Source: CAD feature listing. Evaluate the final solid. Frame: model axes, mm. Round coordinates to 2 decimals unless told otherwise and drop trailing zeros. Order: outer loops, then holes, each group sorted by start corner. A loop starts at its lowest first (then second) coordinate and runs counter-clockwise, first axis right, second up. Notation, with made-up numbers: (20, 81.5) -> (29, 81.5) arc R21 ccw to (29, 93.5) -> close; hole circle Ø10 at (38, 28.25). An arc over 180 degrees is marked (long way). Write item = value, one per line. Start each with the question number.
(1) Cut plane B-B on y = 1781.5. Return the cut outline in (x, z).
(2) Cut plane A-A on x = 27. Return the cut outline in (y, z), then the cut area to 3 significant figures.
(3) Ray query, line 1 (X direction, y = 1627.5, z = 101); line 2 (X direction, y = 1532, z = -3.5); line 3 (Y direction, x = 211, z = 3.5). Return the intervals inside material, ascending.
(4) Contact query for flat-ended pins moving along their axis: pin 1 Ø8 at (y, z) = (701, 21) entering from +X; pin 2 Ø1 at (x, z) = (488.5, 20) entering from -Y (3 decimals); pin 3 Ø2 at (x, z) = (18.5, -0.5) entering from -Y. Output: stop coordinate, or through.
from build123d import *

# Parameters (mm, degrees)
F2_R = 19.05


with BuildPart() as f7:
    # F7: sweep along a path in F0, F4, F0, F4, F0, F6, F0, F6, F0
    with BuildLine(Plane.XY) as f7_path:
        Line((-609.6, 203.2), (-609.6, 0))
    with BuildLine(Plane.YZ.offset(-609.6)) as f7_path_2:
        Line((203.2, 0), (322.2318041258, 119.0318041258))
        Line((322.2318041258, 119.0318041258), (490.5681958742, 119.0318041258))
        Line((490.5681958742, 119.0318041258), (609.6, 0))
    with BuildLine(Plane.XY) as f7_path_3:
        Line((-609.6, 1524), (-609.6, 609.6))
    with BuildLine(Plane.YZ.offset(-609.6)) as f7_path_4:
        Line((1524, 0), (1643.0318041258, 119.0318041258))
        Line((1643.0318041258, 119.0318041258), (1811.3681958742, 119.0318041258))
        Line((1811.3681958742, 119.0318041258), (1930.4, 0))
        Line((1930.4, 0), (2133.6, 0))
    with BuildLine(Plane.XY) as f7_path_5:
        Line((-609.6, 2133.6), (609.6, 2133.6))
        Line((609.6, 2133.6), (609.6, 1930.4))
    with BuildLine(Plane.YZ.offset(609.6)) as f7_path_6:
        Line((1930.4, 0), (1811.3681958742, 119.0318041258))
        Line((1811.3681958742, 119.0318041258), (1643.0318041258, 119.0318041258))
        Line((1643.0318041258, 119.0318041258), (1524, 0))
    with BuildLine(Plane.XY) as f7_path_7:
        Line((609.6, 609.6), (609.6, 1524))
    with BuildLine(Plane.YZ.offset(609.6)) as f7_path_8:
        Line((609.6, 0), (490.5681958742, 119.0318041258))
        Line((490.5681958742, 119.0318041258), (322.2318041258, 119.0318041258))
        Line((322.2318041258, 119.0318041258), (203.2, 0))
    with BuildLine(Plane.XY) as f7_path_9:
        Line((609.6, 203.2), (609.6, 0))
        Line((609.6, 0), (-609.6, 0))
    # F2 (on plane+point) → F7 (sweep)
    with BuildSketch(Plane.XZ):
        with Locations((-609.6, 0)):
            Circle(F2_R)
    sweep(path=f7_path.line + f7_path_2.line + f7_path_3.line + f7_path_4.line + f7_path_5.line + f7_path_6.line + f7_path_7.line + f7_path_8.line + f7_path_9.line, transition=Transition.RIGHT)


solid = f7.part
Evaluation:
q1.outline = circle Ø38.1 at (-609.6, 119.03); circle Ø38.1 at (609.6, 119.03)
q2.outline = circle Ø38.1 at (0, 0); circle Ø38.1 at (2133.6, 0)
q2.area = 2,280 mm^2
q3.line_1 = -628.57 to -590.63, 590.63 to 628.57
q3.line_2 = -626.83 to -592.37, 592.37 to 626.83
q3.line_3 = -18.73 to 18.73, 2114.87 to 2152.33
q4.pin_1 = 618.2
q4.pin_2 = through
q4.pin_3 = -19.05
